Work out the finished part from the listing and answer in its coordinate system (mm). A direction names the side the tool comes from. Coordinates: 2 decimals unless noted, no trailing zeros. Write each loop counter-clockwise with the first axis right and the second up, starting at its lowest first coordinate (ties: lowest second). Pieces come first, ordered by that corner, then holes. Notation, with made-up numbers: (-16.5, 54) - (6.5, 54) arc R18 cw to (6.5, 61) - close; hole circle Ø1 at (10, -7). An arc over 180 degrees is marked (long way). One line per item, written item: value.
```python
from build123d import *

# Parameters (mm, degrees)
CHAMFER1_SIZE      = 0.8
CUT_EXTRUDE1_DEPTH = 6


with BuildPart() as part:
    # Sketch1 → Revolve1 (revolve)
    with BuildSketch(Plane(origin=(0, 0, 0), x_dir=(0, 0, -1), z_dir=(1, 0, 0))):
        Polygon((0, 0), (0, 6.5), (0.53, 7.417986928), (8.53, 7.417986928), (9.06, 6.5), (9.06, 4), (39.06, 4), (39.06, 0), align=None)
    revolve(axis=Axis((0, 0, 0), (0, 0, -1)))

    # Chamfer1
    chamfer1_edges = [part.edges().sort_by_distance(p)[0] for p in [
        (0, -4, -39.06),
    ]]
    chamfer(chamfer1_edges, length=CHAMFER1_SIZE)

    # Sketch2 → Cut-Extrude1 (cut)
    with BuildSketch(Plane.XY):
        Polygon((-3.25, 1.876388375), (-3.25, -1.876388375), (0, -3.75277675), (3.25, -1.876388375), (3.25, 1.876388375), (0, 3.75277675), align=None)
    extrude(amount=-CUT_EXTRUDE1_DEPTH, mode=Mode.SUBTRACT)

    # Sketch3 → Cut-Revolve2 (revolve, cut)
    with BuildSketch(Plane(origin=(0, 0, 0), x_dir=(0, 0, -1), z_dir=(1, 0, 0))):
        Polygon((6, 0), (6, 3.75277675), (8.166666667, 0), align=None)
    revolve(axis=Axis((0, 0, 0), (0, 0, -1)), mode=Mode.SUBTRACT)


solid = part.part
```
Item 1: Consider probe 1 along Z at (x, y) = (3.5, -2.5); probe 2 along Z at (x, y) = (-2.25, 2.5); probe 3 along X at (y, z) = (1.5, -1.5). Determine where each line is inside the solid, lowest interval first.
Evaluation:
probe 1: z = -9.06 to 0
probe 2: z = -38.9 to -6.22, -6 to 0
probe 3: x = -7.26 to -3.25, 3.25 to 7.26
Item 2: Section B-B, the plane z = -31 is taken. Determine the outline of the cut face in (x, y), then the cut area to 3 significant figures.
Evaluation:
outline: circle Ø8 at (0, 0)
area: 50.3 mm2
Item 3: Given pin 1 (4 mm diameter, centred on y = -0.5, z = -2.5, fed in from +X); pin 2 (1.5 mm diameter, centred on y = 0, z = -17.5, fed in from -X); pin 3 (3 mm diameter, centred on x = 3, z = -12.5, fed in from -Y); pin 4 (6 mm diameter, centred on x = 2, z = -28.5, fed in from +Y), each flat-ended and moving along its own axis, determine where each tip first touches the part or whether it passes through.
Evaluation:
pin 1: stops at x = 7.42
pin 2: stops at x = -4
pin 3: stops at y = -3.71
pin 4: stops at y = 4
Item 4: Determine the mould class of faces 5 (the face through (3.25, 0, -3)), 6 (the face through (2, 3, 0)), 7 (the face through (-3.905, -0.867, -23.864)) for opening direction X: +X half, -X half, draft (parallel to the pull), parting line (faces both ways), or undercut.
Evaluation:
face 5: undercut
face 6: draft
face 7: parting line
Item 5: Which of the six approach directions +Z, -Z, +X, -X, +Y, -Y give full straight-line access (tool end or side, diameter ignored) to faces 1 (the face through (3, 3, -9.06)), 2 (the face through (0, 0, -39.06)), 3 (the face through (-1.7, 3, -6)), 4 (the face through (-1.6, 2.83, -2.96))?
Evaluation:
face 1: -Z
face 2: -Z, +X, -X, +Y, -Y
face 3: none
face 4: +Z
Item 6: Section A-A, the plane z = -4.5 is taken. Determine the outline of the cut face in (x, y).
Evaluation:
outline: circle Ø14.84 at (0, 0); hole (-3.25, -1.88) - (0, -3.75) - (3.25, -1.88) - (3.25, 1.88) - (0, 3.75) - (-3.25, 1.88) - close
